```python
from build123d import *

# Parameters (mm, degrees)
SKETCH_1_R          = 9.5
EXTRUDE_1_DEPTH     = 25
FILLET_1_R          = 2
HOLE_WIZARD_1_D     = 8
HOLE_WIZARD_1_DEPTH = 12.5
HOLE_WIZARD_2_D     = 5


with BuildPart() as part:
    # Sketch 1 → Extrude 1 (new body)
    with BuildSketch(Plane(origin=(0, 0, 0), x_dir=(1, 0, 0), z_dir=(0, 1, 0))):
        with Locations(Location((0, 0, 0), (0, 0, 270))):
            Circle(SKETCH_1_R)
    extrude(amount=EXTRUDE_1_DEPTH)

    # Fillet 1
    fillet_1_edges = [part.edges().sort_by_distance(p)[0] for p in [
        (0, 0, -9.5),
        (0, 25, -9.5),
    ]]
    fillet(fillet_1_edges, radius=FILLET_1_R)

    # Hole Wizard 1
    with Locations(Plane(origin=(0, 25, 0), x_dir=(1, 0, 0), z_dir=(0, 1, 0))):
        with Locations((0, 0)):
            Hole(HOLE_WIZARD_1_D / 2, depth=HOLE_WIZARD_1_DEPTH)

    # Hole Wizard 2 (through all)
    with Locations(Plane(origin=(0, 0, 0), x_dir=(-1, 0, 0), z_dir=(0, -1, 0))):
        with Locations((0, 0)):
            Hole(HOLE_WIZARD_2_D / 2)


solid = part.part
```
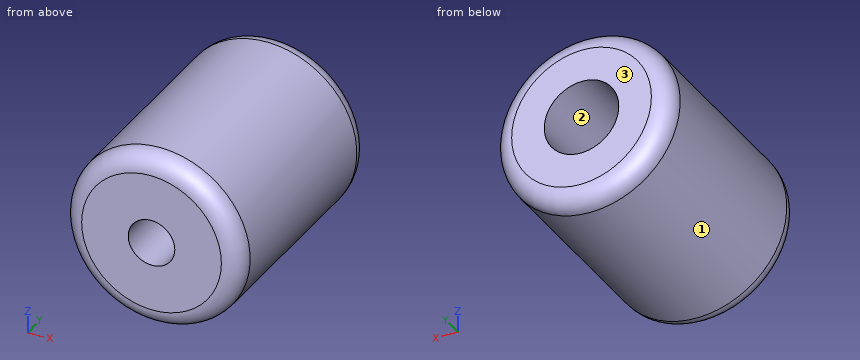
Can you work these out from the model? Positions are in its coordinate system, mm. Face numbers are marked on the shaded views. Coordinates: 2 decimals unless noted, no trailing zeros. Loops run counter-clockwise (first coordinate to the right, second up) from the corner with the lowest first, then second, coordinate; pieces in that order, holes last. Notation, with made-up numbers: (39, -6) -> (51, -6) arc R34 ccw to (51, 25) -> close; hole circle Ø11 at (51, 34.25). An arc over 180 degrees is marked (long way). Put each result on its own line as item: value. Start each with the question number.
Q1. Thinking about a two-plate mould opening in Z: for the marked faces 1, 2 and 3, which applies, pulls with the +Z half, pulls with the -Z half, needs draft (parallel to the pull), parting line crosses it, or undercut?
Q2. If I drill on line 1 (Z direction, x = 0.5, y = 10); line 2 (Y direction, x = 1.75, z = 2); line 3 (X direction, y = 21, z = -0.5), over which ranges is the centre line in solid material (lowest first)? Write a range as [from, to].
Q3. I want a section at B-B (x = 0). Write out the boundary of the cut face in (y, z).
Q4. I want a section at C-C (y = 8.25). Write out the boundary of the cut face in (x, z).
Q5. I want a section at A-A (z = 0). Write out the boundary of the cut face in (x, y), plus the area to 3 significant figures.
Q6. I want a section at D-D (y = 14). Write out the boundary of the cut face in (x, z).
Q7. I'm going to push flat-ended pins straight in: P1, Ø5, axis at y = 13.5, z = -6, coming from the -X side; P2, Ø5, axis at y = 16.5, z = 1, coming from the -X side; P3, Ø1.5, axis at x = -1, y = 4, coming from the +Z side; P4, Ø4, axis at x = -1.5, z = 1, coming from the +Y side. Where does each tip first touch, or does it pass through?
Taken from the geometry:
1. face 1: parting line crosses it
1. face 2: undercut
1. face 3: needs draft
2. line 1: z = [-9.49, -2.45], [2.45, 9.49]
2. line 2: y = [0, 12.5]
2. line 3: x = [-9.49, -3.97], [3.97, 9.49]
3. outline: (0, -7.5) arc R2 ccw to (2, -9.5) -> (23, -9.5) arc R2 ccw to (25, -7.5) -> (25, -4) -> (12.5, -4) -> (12.5, -2.5) -> (0, -2.5) -> close; (0, 2.5) -> (12.5, 2.5) -> (12.5, 4) -> (25, 4) -> (25, 7.5) arc R2 ccw to (23, 9.5) -> (2, 9.5) arc R2 ccw to (0, 7.5) -> close
4. outline: circle Ø19 at (0, 0); hole circle Ø5 at (0, 0)
5. outline: (-9.5, 2) arc R2 ccw to (-7.5, 0) -> (-2.5, 0) -> (-2.5, 12.5) -> (-4, 12.5) -> (-4, 25) -> (-7.5, 25) arc R2 ccw to (-9.5, 23) -> close; (2.5, 0) -> (7.5, 0) arc R2 ccw to (9.5, 2) -> (9.5, 23) arc R2 ccw to (7.5, 25) -> (4, 25) -> (4, 12.5) -> (2.5, 12.5) -> close
5. area: 309 mm2
6. outline: circle Ø19 at (0, 0); hole circle Ø8 at (0, 0)
7. P1: stops at x = -8.83
7. P2: stops at x = -9.5
7. P3: stops at z = 9.5
7. P4: stops at y = 12.5
